Part model, mm, in its own coordinate system. A direction names the side the tool comes from. Coordinates: 2 decimals unless noted, no trailing zeros. Write each loop counter-clockwise with the first axis right and the second up, starting at its lowest first coordinate (ties: lowest second). Pieces come first, ordered by that corner, then holes. Notation, with made-up numbers: (-24.75, 43) - (-14.75, 43) arc R33 cw to (-14.75, 77) - close; hole circle Ø3 at (36, 76.25). An arc over 180 degrees is marked (long way). Use a Markdown table: item, result.
Autodesk Inventor part; units mm, degrees
ref_plane "YZ Plane" through (0, 0, 0) normal (1, 0, 0) x (0, 1, 0)
ref_plane "XZ Plane" through (0, 0, 0) normal (0, 1, 0) x (-1, 0, 0)
ref_plane "XY Plane" through (0, 0, 0) normal (0, 0, 1) x (1, 0, 0)
sketch "Sketch1" plane through (0, 0, 0) normal (0, 1, 0) x (-1, 0, 0)
  line L0 (21.336, 6.35) -> (-47.371, 6.35)
  line L1 (-47.371, 6.35) -> (-47.371, -6.35)
  line L2 (-47.371, -6.35) -> (21.336, -6.35)
  line L3 (21.336, -6.35) -> (21.336, 6.35)
  line L4 (-2.54, -2.54) -> (2.54, -2.54)
  line L5 (2.54, -2.54) -> (2.54, 2.54)
  line L6 (2.54, 2.54) -> (-2.54, 2.54)
  line L7 (-2.54, 2.54) -> (-2.54, -2.54)
  line L8 (-2.54, -2.54) -> (2.54, 2.54) construction
  line L9 (2.54, -2.54) -> (-2.54, 2.54) construction
  line L10 (-10.668, 2.54) -> (-15.748, 2.54)
  line L11 (-15.748, 2.54) -> (-15.748, -2.54)
  line L12 (-15.748, -2.54) -> (-10.668, -2.54)
  line L13 (-10.668, -2.54) -> (-10.668, 2.54)
  line L14 (-10.668, 2.54) -> (-15.748, -2.54) construction
  line L15 (-15.748, 2.54) -> (-10.668, -2.54) construction
  line L16 (-23.876, 2.54) -> (-28.956, 2.54)
  line L17 (-28.956, 2.54) -> (-28.956, -2.54)
  line L18 (-28.956, -2.54) -> (-23.876, -2.54)
  line L19 (-23.876, -2.54) -> (-23.876, 2.54)
  line L20 (-23.876, 2.54) -> (-28.956, -2.54) construction
  line L21 (-28.956, 2.54) -> (-23.876, -2.54) construction
  point P0 (0, 0)
  point P1 (-13.208, 0)
  point P2 (-26.416, 0)
  dimension "d0" = 68.707
  dimension "d1" = 12.7
  dimension "d2" = 5.08
  dimension "d3" = 5.08
  dimension "d4" = 5.08
  dimension "d5" = 5.08
  dimension "d6" = 13.208
  dimension "d7" = 13.208
  dimension "d8" = 6.35
  dimension "d9" = 21.336
  dimension "d37" = 5.08
  dimension "d38" = 5.08
extrude "Extrusion1" add sketch "Sketch1" along normal blind 2.286
sketch "Sketch2" plane through (0, 2.286, 0) normal (0, 1, 0) x (1, 0, 0)
  line L0 (-21.336, 6.35) -> (-21.336, -6.35)
  circle A0 centre (-14.986, 0) radius 4.0259
  point P0 (0, 0)
  dimension "d12" = 6.35
  dimension "d13" = 8.0518
extrude "Extrusion2" add sketch "Sketch2" along normal blind 5.207
sketch "Sketch3" plane through (-14.986, 7.493, 0) normal (0, 1, 0) x (1, 0, 0)
  circle A0 centre (0, 0) radius 3.2385
  point P0 (14.986, 0)
  dimension "d16" = 6.477
extrude "Extrusion3" cut sketch "Sketch3" against normal blind 0.7874
sketch "Sketch4" plane through (0, 0, 0) normal (0, -1, 0) x (1, 0, 0)
  circle A0 centre (-14.986, 0) radius 3.2385
  circle A1 centre (-14.986, 0) radius 3.2385
  point P0 (0, 0)
  dimension "d39" = 6.477
extrude "Extrusion4" cut sketch "Sketch4" against normal blind 0.7874
sketch "Sketch5" plane through (-14.986, 6.7056, 0) normal (0, 1, 0) x (1, 0, 0)
  circle A0 centre (0, 0) radius 2.5781
  point P0 (14.986, 0)
  dimension "d21" = 5.1562
extrude "Extrusion5" cut sketch "Sketch5" against normal through all
sketch "Sketch6" plane through (0, 2.286, 0) normal (0, 1, 0) x (1, 0, 0)
  line L0 (47.371, -6.35) -> (47.371, 6.35)
  circle A0 centre (41.021, 0) radius 4.0259
  point P0 (0, 0)
  dimension "d24" = 6.35
  dimension "d25" = 8.0518
extrude "Extrusion6" add sketch "Sketch6" along normal blind 5.207
sketch "Sketch7" plane through (41.021, 7.493, 0) normal (0, 1, 0) x (1, 0, 0)
  circle A0 centre (0, 0) radius 3.2385
  point P0 (-41.021, 0)
  dimension "d28" = 6.477
extrude "Extrusion7" cut sketch "Sketch7" against normal blind 0.7874
sketch "Sketch8" plane through (0, 0, 0) normal (0, -1, 0) x (1, 0, 0)
  circle A0 centre (41.021, 0) radius 3.2385
  circle A1 centre (41.021, 0) radius 3.2385
  point P0 (0, 0)
  dimension "d40" = 6.477
extrude "Extrusion8" cut sketch "Sketch8" against normal blind 0.7874
sketch "Sketch9" plane through (41.021, 6.7056, 0) normal (0, 1, 0) x (1, 0, 0)
  circle A0 centre (0, 0) radius 2.5781
  point P0 (-41.021, 0)
  dimension "d33" = 5.1562
extrude "Extrusion9" cut sketch "Sketch9" against normal through all
fillet "Fillet1" radius 6.35 4 edges at (47.371, 1.143, 6.35) (47.371, 1.143, -6.35) (-21.336, 1.143, 6.35) (-21.336, 1.143, -6.35)
sketch "Sketch12" plane through (-14.986, 7.493, 0) normal (0, 1, 0) x (1, 0, 0)
  circle A0 centre (0, 0) radius 4.0259
  line L0 (0, 0) -> (4.0259, 0) construction
  line L1 (0, 0) -> (4.0259, 0) construction
  circle A1 centre (0, 0) radius 3.2385
  line L2 (-3.1893, 0.5624) -> (-3.9647, 0.6991)
  line L3 (-3.1893, -0.5624) -> (-3.9647, -0.6991)
  arc A2 (-3.1893, 0.5624) -> (-3.1893, -0.5624) centre (0, 0) ccw
  arc A3 (-3.9647, 0.6991) -> (-3.9647, -0.6991) centre (0, 0) ccw
  point P0 (14.986, 0)
  point P1 (-2.9392, 0.5183)
extrude "Extrusion11" cut sketch "Sketch12" against normal blind 0.762 contours L2 A1 L3 A0 picked at (-3.7571, 0.0628)
properties part number "VexLegoMountThick2"
Item 1: Band-saw the part on C-C, the plane x = 43. Give the cut face in (y, z).
From the geometry:
| item | result |
|---|---|
| outline | (0, -6.03) - (2.29, -6.03) - (2.29, -3.51) - (7.49, -3.51) - (7.49, -2.56) - (6.71, -2.56) - (6.71, -1.65) - (0.79, -1.65) - (0.79, -2.56) - (0, -2.56) - close; (0, 2.56) - (0.79, 2.56) - (0.79, 1.65) - (6.71, 1.65) - (6.71, 2.56) - (7.49, 2.56) - (7.49, 3.51) - (2.29, 3.51) - (2.29, 6.03) - (0, 6.03) - close |
Item 2: Band-saw the part on D-D, the plane x = 7. Give the cut face in (y, z).
From the geometry:
| item | result |
|---|---|
| outline | (0, -6.35) - (2.29, -6.35) - (2.29, 6.35) - (0, 6.35) - close |
Item 3: Two-plate mould, pull along X, no slides. Class faces 1 (the face through (45.6, 1.2, -4.4)), 2 (the face through (13, 1, 2.54)), 3 (the face through (-13, 7.493, -3)): pulls with the +X half, pulls with the -X half, needs draft (parallel to the pull), parting line crosses it, or undercut.
From the geometry:
| item | result |
|---|---|
| face 1 | pulls with the +X half |
| face 2 | undercut |
| face 3 | needs draft |
Item 4: Drop flat-ended pins along their axis: P1, Ø1, axis at x = -10, y = 3, coming from the -Z side; P2, Ø2, axis at x = -8, z = -1.5, coming from the +Y side; P3, Ø1.9, axis at x = 39.5, z = -1, coming from the -Y side; P4, Ø1.5, axis at y = 5.5, z = -1.5, coming from the +X side. Give the stop position or say it passes through.
From the geometry:
| item | result |
|---|---|
| P1 | through |
| P2 | y = 2.29 |
| P3 | y = 0.79 |
| P4 | x = 44.98 |
Item 5: Band-saw the part on B-B, the plane y = 3.25. Give the cut face in (x, z), then the cut area to 3 significant figures.
From the geometry:
| item | result |
|---|---|
| outline | circle Ø8.05 at (-14.99, 0); circle Ø8.05 at (41.02, 0); hole circle Ø5.16 at (-14.99, 0); hole circle Ø5.16 at (41.02, 0) |
| area | 60.1 mm^2 |
Item 6: Drill centre lines: probe 1 along X at (y, z) = (6.95, 0); probe 2 along X at (y, z) = (2.2, 0); probe 3 along X at (y, z) = (3.8, 0). Where is each one in solid material? Low to high.
From the geometry:
| item | result |
|---|---|
| probe 1 | -11.75 to -10.96, 37 to 37.78, 44.26 to 45.05 |
| probe 2 | -21.34 to -17.56, -12.41 to -2.54, 2.54 to 10.67, 15.75 to 23.88, 28.96 to 38.44, 43.6 to 47.37 |
| probe 3 | -19.01 to -17.56, -12.41 to -10.96, 37 to 38.44, 43.6 to 45.05 |
Item 7: Which spindle directions (+Z, -Z, +X, -X, +Y, -Y) get a long thin tool onto all of the face, cutting with end or side? Do faces 4 (the face through (-11.897, 7.105, -0.973)), 5 (the face through (-11.994, 0.388, -1.24)), 6 (the face through (26, 1, 2.54)). Say none if no direction does.
From the geometry:
| item | result |
|---|---|
| face 4 | +Y |
| face 5 | -Y |
| face 6 | +Y, -Y |
Item 8: Band-saw the part on A-A, the plane x = 14. Give the cut face in (y, z).
From the geometry:
| item | result |
|---|---|
| outline | (0, -6.35) - (2.29, -6.35) - (2.29, -2.54) - (0, -2.54) - close; (0, 2.54) - (2.29, 2.54) - (2.29, 6.35) - (0, 6.35) - close |
